CAD build for the part. Positions are in the model's coordinates, mm. A direction names the side the tool comes from. Round coordinates to 2 decimals unless told otherwise and drop trailing zeros. Loops run counter-clockwise (first coordinate to the right, second up) from the corner with the lowest first, then second, coordinate; pieces in that order, holes last.
from build123d import *

# Parameters (mm, degrees)
SKETCH1_W           = 560
SKETCH1_H           = 120
SKETCH1_W_2         = 500
SKETCH1_H_2         = 60
BOSS_EXTRUDE1_DEPTH = 15
CUT_EXTRUDE1_DEPTH  = 250


with BuildPart() as part:
    # Sketch1 → Boss-Extrude1 (new, symmetric)
    with BuildSketch(Plane.XY):
        Rectangle(SKETCH1_W, SKETCH1_H)
        Rectangle(SKETCH1_W_2, SKETCH1_H_2, mode=Mode.SUBTRACT)
    extrude(amount=BOSS_EXTRUDE1_DEPTH, both=True)

    # Sketch2 → Cut-Extrude1 (cut, symmetric)
    with BuildSketch(Plane(origin=(0, 0, 0), x_dir=(0, 0, -1), z_dir=(1, 0, 0))):
        Polygon((-4, 31), (-6.5, 30), (6.5, 30), (4, 31), (4, 32), (7.5, 32), (7.5, 36), (0, 40), (-7.5, 36), (-7.5, 32), (-4, 32), align=None)
        Polygon((-6.5, -30), (6.5, -30), (4, -31), (4, -32), (7.5, -32), (7.5, -36), (0, -40), (-7.5, -36), (-7.5, -32), (-4, -32), (-4, -31), align=None)
    extrude(amount=CUT_EXTRUDE1_DEPTH, both=True, mode=Mode.SUBTRACT)


solid = part.part
Item 1: Cut at A-A (y = 12). List the corners of the cut face in (x, z).
Verdict:
outline: (-280, -15) - (-250, -15) - (-250, 15) - (-280, 15) - close; (250, -15) - (280, -15) - (280, 15) - (250, 15) - close
Item 2: 3-axis set-ups, long thin cutter, end or side, ignore diameter. For faces 1 (the flat face through (-250, -1, 0)), 2 (the flat face through (280, -1, 0)): which of +Z, -Z, +X, -X, +Y, -Y reach the whole face in a straight line?
Verdict:
face 1: none
face 2: +Z, -Z, +X, +Y, -Y
Item 3: Mould opens along Y. For faces 3 (the flat face through (-280, -1, 0)), 4 (the flat face through (250, -1, 0)), 5 (the flat face through (-4, 60, 0)) say: released by +Y, released by -Y, zero draft, split by the parting line, or undercut.
Verdict:
face 3: zero draft
face 4: undercut
face 5: released by +Y
Item 4: Wall check: L1, parallel to X at y = -18, z = 11.25; L2, parallel to Y at x = -239, z = 9.25; L3, parallel to Y at x = 177.5, z = -5.75. Give the ranges that are in metal, low to high.
Verdict:
L1: x = -280 to -250, 250 to 280
L2: y = -60 to -30, 30 to 60
L3: y = -60 to -36.93, -32 to -30.3, 30.3 to 32, 36.93 to 60
